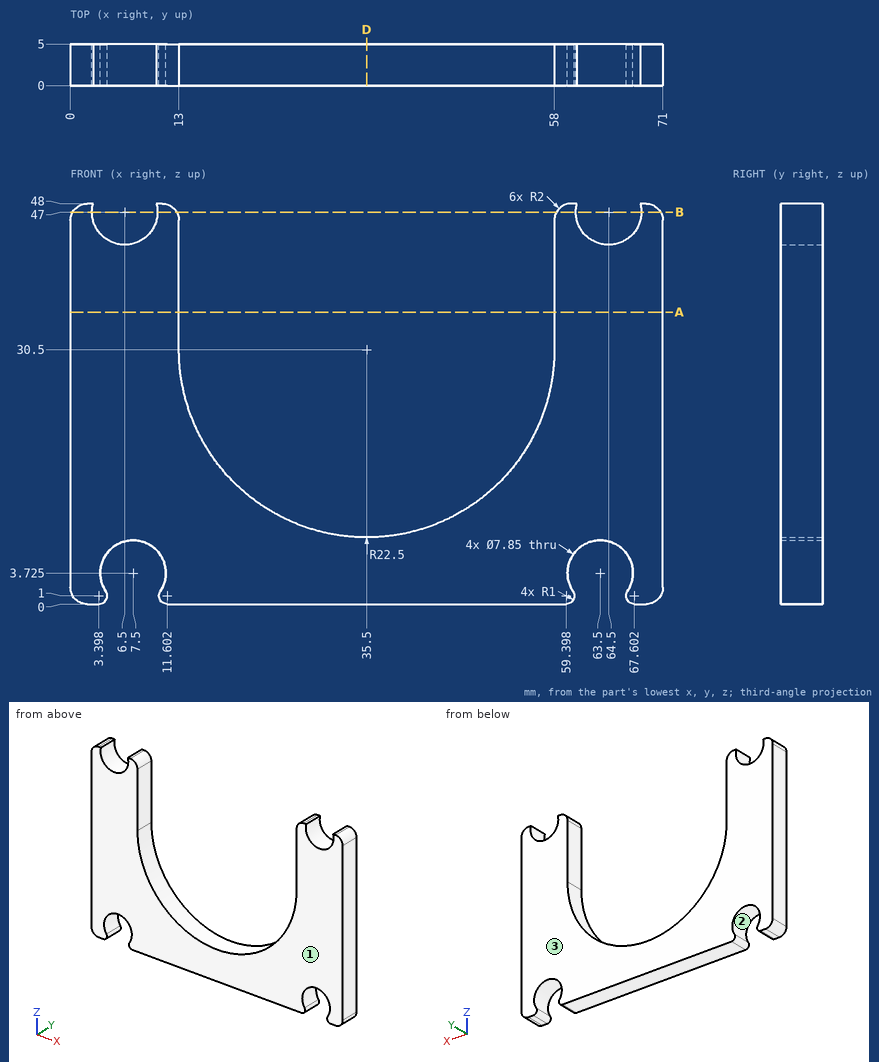
Print and shaded views of the part. All mm, measured from the part's lowest x, y and z. Round coordinates to 2 decimals unless told otherwise and drop trailing zeros. Loops run counter-clockwise (first coordinate to the right, second up) from the corner with the lowest first, then second, coordinate; pieces in that order, holes last. Notation, with made-up numbers: M 73.25,-22 L 109.25,-22 A11 ccw 109.25,-18 Z; hole C 44.25,-37 d5. An arc over 180 degrees is marked long. One line per question, with ' | ' between items.
1) Band-saw the part on A-A (z = 35). Give the cut face in (x, y), then the cut area to 3 significant figures.
Solved:
outline: M 0,0 L 13,0 L 13,5 L 0,5 Z; M 58,0 L 71,0 L 71,5 L 58,5 Z | area: 130 mm²
2) Band-saw the part on D-D (x = 35.5). Give the cut face in (y, z).
Solved:
outline: M 0,0 L 5,0 L 5,8 L 0,8 Z
3) Mould opens along Y. For the marked faces 1, 2 and 3 say: +Y half, -Y half, draft (parallel to the pull), parting line (faces both ways), or undercut.
Solved:
face 1: -Y half | face 2: draft | face 3: +Y half
4) Drill centre lines: line 1 along X through (y, z) = (4.45, 6); line 2 along X through (y, z) = (3.4, 6.5) (1 decimal); line 3 along X through (y, z) = (1.15, 47) (1 decimal). Where is each one in solid material? Low to high.
Solved:
line 1: x = 0 to 4.3, 10.7 to 60.3, 66.7 to 71 | line 2: x = 0 to 4.7, 10.3 to 60.7, 66.3 to 71 | line 3: x = 0.3 to 2.6, 10.4 to 12.7, 58.3 to 60.6, 68.4 to 70.7
5) Band-saw the part on B-B (z = 47). Give the cut face in (x, y) (1 decimal).
Solved:
outline: M 0.3,0 L 2.6,0 L 2.6,5 L 0.3,5 Z; M 10.4,0 L 12.7,0 L 12.7,5 L 10.4,5 Z; M 58.3,0 L 60.6,0 L 60.6,5 L 58.3,5 Z; M 68.4,0 L 70.7,0 L 70.7,5 L 68.4,5 Z
